The model under review builds one solid part; all positions refer to its coordinate system, in mm. A direction names the side the tool comes from. Coordinates: 2 decimals unless noted, no trailing zeros. Loops run counter-clockwise (first coordinate to the right, second up) from the corner with the lowest first, then second, coordinate; pieces in that order, holes last. Notation, with made-up numbers: M 15,71.25 L 64,71.25 A16 cw 64,78.25 Z; hole C 7.25,-28 d6. An arc over 180 degrees is marked long. Use CSV: the item, a comma, the result in double quotes. Start each with the question number.
1. Draft analysis for pull direction Z (two halves, no side actions). For faces 6 (the flat face through (-5, 0, 38)), 7 (the flat face through (2, 0, 42.5)), 8 (the flat face through (1.6, 5, 39.5)), state which applies: +Z half, -Z half, draft (parallel to the pull), parting line (faces both ways), or undercut.
2. Add section B-B, the plane y = 0. State how many separate pieces and enclosed holes the cut face has, then the cut area to 3 significant figures.
3. Clearance check with flat-ended pins moving along their axes: P1, Ø2.5, axis at x = 6, z = 24, coming from the +Y side; P2, Ø0.9, axis at x = -7, z = 24, coming from the +Y side; P3, Ø12, axis at y = -9.5, z = 16.5, coming from the -X side. State where each tip first meets the part, or that it passes through.
4. For L1, parallel to Z at x = -0.75, y = -6.25; L2, parallel to Y at x = 0, z = 10.75; L3, parallel to Z at x = -3.25, y = -7.5, list the stretches that pass through material, from the lowest coordinate up.
5. Add section A-A, the plane z = 6.5. Write out the cut boundary in (x, y), then the cut area to 3 significant figures.
6. Tool access review of faces 1 (the cylindrical face through (0, -2, 10)), 2 (the cylindrical face through (3.233, -1.341, 28.232)), 3 (the flat face through (6, 1.5, 24)), 4 (the flat face through (1, -4, 35)), 5 (the flat face through (1, 6, 42)): name each direction out of +Z, -Z, +X, -X, +Y, -Y from which nothing blocks a thin tool from reaching the whole face with its end or side.
7. Add section C-C, the plane y = -11. Write out the cut boundary in (x, z), then the cut area to 3 significant figures.
8. Add section D-D, the plane x = 12. Write out the cut boundary in (y, z).
from build123d import *

# Parameters (mm, degrees)
F0_R          = 14
F0_R_2        = 12.5
F0_R_3        = 3.5
F0_R_4        = 2
F1_DEPTH      = 2.5
F2_DEPTH      = 15
F3_R          = 14
F3_R_2        = 2
F4_DEPTH      = 2.5
F5_R          = 9
F5_R_2        = 7.5
F5_R_3        = 3.5
F5_R_4        = 2
F6_DEPTH      = 25
F8_DEPTH      = 25
F8_DEPTH_BACK = 25
F9_W          = 8
F9_H          = 14.2362220213
F10_DEPTH     = 10
F11_DEPTH     = 25
F13_DEPTH     = 3
F14_DEPTH     = 2.5
F15_START     = 9.5
F15_DEPTH     = 2.5
F16_SIZE2     = 1.99999
F16_SIZE      = 1.99999


# Not quite as in the source:
# - a fillet or chamfer is up to 0.001 mm smaller than in the source, because OpenCascade refuses the exact size


with BuildPart() as f1:
    # F0 (on Top) → F1 (new body)
    with BuildSketch(Plane.XY):
        Circle(F0_R)
        Circle(F0_R_2, mode=Mode.SUBTRACT)
        Circle(F0_R_2)
        Circle(F0_R_3, mode=Mode.SUBTRACT)
        Circle(F0_R_3)
        Circle(F0_R_4, mode=Mode.SUBTRACT)
    extrude(amount=-F1_DEPTH)

    # F0 (on Top) → F2 (join)
    with BuildSketch(Plane.XY):
        Circle(F0_R)
        Circle(F0_R_2, mode=Mode.SUBTRACT)
        Circle(F0_R_3)
        Circle(F0_R_4, mode=Mode.SUBTRACT)
    extrude(amount=F2_DEPTH)

    # F3 (on face) → F4 (join)
    with BuildSketch(Plane.XY.offset(15)):
        Circle(F3_R)
        Circle(F3_R_2, mode=Mode.SUBTRACT)
    extrude(amount=F4_DEPTH)

    # F5 (on face) → F6 (join)
    with BuildSketch(Plane.XY.offset(17.5)):
        Circle(F5_R)
        Circle(F5_R_2, mode=Mode.SUBTRACT)
        Circle(F5_R_2)
        Circle(F5_R_3, mode=Mode.SUBTRACT)
        Circle(F5_R_3)
        Circle(F5_R_4, mode=Mode.SUBTRACT)
        Circle(F5_R_4)
    extrude(amount=F6_DEPTH)

    # F7 (on Right) → F8 (cut, two sides)
    with BuildSketch(Plane.YZ) as f8_sk:
        Polygon((-6, 40.5), (-6, 42.5), (-9, 42.5), (-9, 32.5), (-4, 32.5), (-4, 40.5), align=None)
        Polygon((9, 42.5), (6, 42.5), (6, 40.5), (4, 40.5), (4, 32.5), (9, 32.5), align=None)
    extrude(amount=F8_DEPTH, mode=Mode.SUBTRACT)
    extrude(f8_sk.sketch, amount=-F8_DEPTH_BACK, mode=Mode.SUBTRACT)

    # F9 (on face) → F10 (cut)
    with BuildSketch(Plane.XY.offset(42.5)):
        with Locations((-9, 0)):
            Rectangle(F9_W, F9_H)
    extrude(amount=-F10_DEPTH, mode=Mode.SUBTRACT)

    # F0 (on Top) → F11 (cut)
    with BuildSketch(Plane.XY):
        Circle(F0_R_4)
    extrude(amount=F11_DEPTH, mode=Mode.SUBTRACT)

    # F12 (on face) → F13 (cut)
    with BuildSketch(Plane(origin=(0, 0, 25), x_dir=(1, 0, 0), z_dir=(0, 0, -1))):
        Polygon((2.5980762114, -1.5), (23.6776883676, -1.5), (23.6776883676, 1.5), (2.5980762114, 1.5), (1.7320508076, 0), align=None)
        Polygon((13.1378822895, -19.7554796292), (2.5980762114, -1.5), (0.8660254038, -1.5), (0, -3), (10.5398060781, -21.2554796292), align=None)
        Polygon((0.8660254038, -1.5), (2.5980762114, -1.5), (1.7320508076, 0), align=None)
        Polygon((0, -3), (0.8660254038, -1.5), (-0.8660254038, -1.5), align=None)
        Polygon((0.8660254038, 1.5), (1.7320508076, 0), (2.5980762114, 1.5), align=None)
        Polygon((0.8660254038, 1.5), (2.5980762114, 1.5), (13.1378822895, 19.7554796292), (10.5398060781, 21.2554796292), (0, 3), align=None)
        Polygon((0, -3), (-0.8660254038, -1.5), (-2.5980762114, -1.5), (-13.1378822895, -19.7554796292), (-10.5398060781, -21.2554796292), align=None)
        Polygon((-2.5980762114, -1.5), (-0.8660254038, -1.5), (-1.7320508076, 0), align=None)
        Polygon((-0.8660254038, 1.5), (0.8660254038, 1.5), (0, 3), align=None)
        Polygon((-23.6776883676, -1.5), (-2.5980762114, -1.5), (-1.7320508076, 0), (-2.5980762114, 1.5), (-23.6776883676, 1.5), align=None)
        Polygon((-2.5980762114, 1.5), (-1.7320508076, 0), (-0.8660254038, 1.5), align=None)
        Polygon((-2.5980762114, 1.5), (-0.8660254038, 1.5), (0, 3), (-10.5398060781, 21.2554796292), (-13.1378822895, 19.7554796292), align=None)
    extrude(amount=F13_DEPTH, mode=Mode.SUBTRACT)

    # F5 (on face) → F14 (cut)
    with BuildSketch(Plane.XY.offset(17.5)):
        Circle(F5_R_2)
        Circle(F5_R_3, mode=Mode.SUBTRACT)
    extrude(amount=F14_DEPTH, mode=Mode.SUBTRACT)

    # F5 (on face) → F15 (cut)
    with BuildSketch(Plane.XY.offset(17.5).offset(F15_START)):
        Circle(F5_R_2)
        Circle(F5_R_3, mode=Mode.SUBTRACT)
    extrude(amount=F15_DEPTH, mode=Mode.SUBTRACT)

    # F16 (size 2 and 2 in the source; OpenCascade refuses exactly that, so slightly less here)
    f16_edges = [f1.edges().sort_by_distance(p)[0] for p in [
        (1.531129, -4, 40.5),
        (1.531129, 4, 40.5),
    ]]
    chamfer(f16_edges, length=F16_SIZE, length2=F16_SIZE2)


solid = f1.part
Computed:
1,face 6,"draft"
1,face 7,"+Z half"
1,face 8,"undercut"
2,separate pieces,"3"
2,enclosed holes,"6"
2,area,"508 mm^2"
3,P1,"stops at y = 7.31"
3,P2,"stops at y = 6.17"
3,P3,"stops at x = -13.56"
4,L1,"z = -2.5 to 0, 15 to 17.5, 20 to 27, 29.5 to 32.5"
4,L2,"y = -14 to -12.5, -3.5 to -2, 2 to 3.5, 12.5 to 14"
4,L3,"z = -2.5 to 0, 15 to 22, 25 to 32.5"
5,outline,"C 0,0 d28; C 0,0 d7; hole C 0,0 d25; hole C 0,0 d4"
5,area,"151 mm^2"
6,face 1,"-Z"
6,face 2,"none"
6,face 3,"+X, -X"
6,face 4,"+X, -X, -Y"
6,face 5,"+Z, +X, -X, +Y"
7,outline,"M -8.66,-2.5 L 8.66,-2.5 L 8.66,17.5 L -8.66,17.5 Z; hole M -5.94,0 L 5.94,0 L 5.94,15 L -5.94,15 Z"
7,area,"168 mm^2"
8,outline,"M -7.21,-2.5 L 7.21,-2.5 L 7.21,17.5 L -7.21,17.5 Z; hole M -3.5,0 L 3.5,0 L 3.5,15 L -3.5,15 Z"
